Source: three-view drawing plus pictorial views. Frame: mm from the lowest corner of the part. Coordinates: 2 decimals unless noted, no trailing zeros. Order: outer loops, then holes, each group sorted by start corner. A loop starts at its lowest first (then second) coordinate and runs counter-clockwise, first axis right, second up. Notation, with made-up numbers: (21.25, 68.5) - (73.25, 68.5) arc R5 cw to (73.25, 73.5) - close; hole circle Ø3 at (71.25, 84.25). An arc over 180 degrees is marked (long way). Use a Markdown table: item, result. Add a question column.
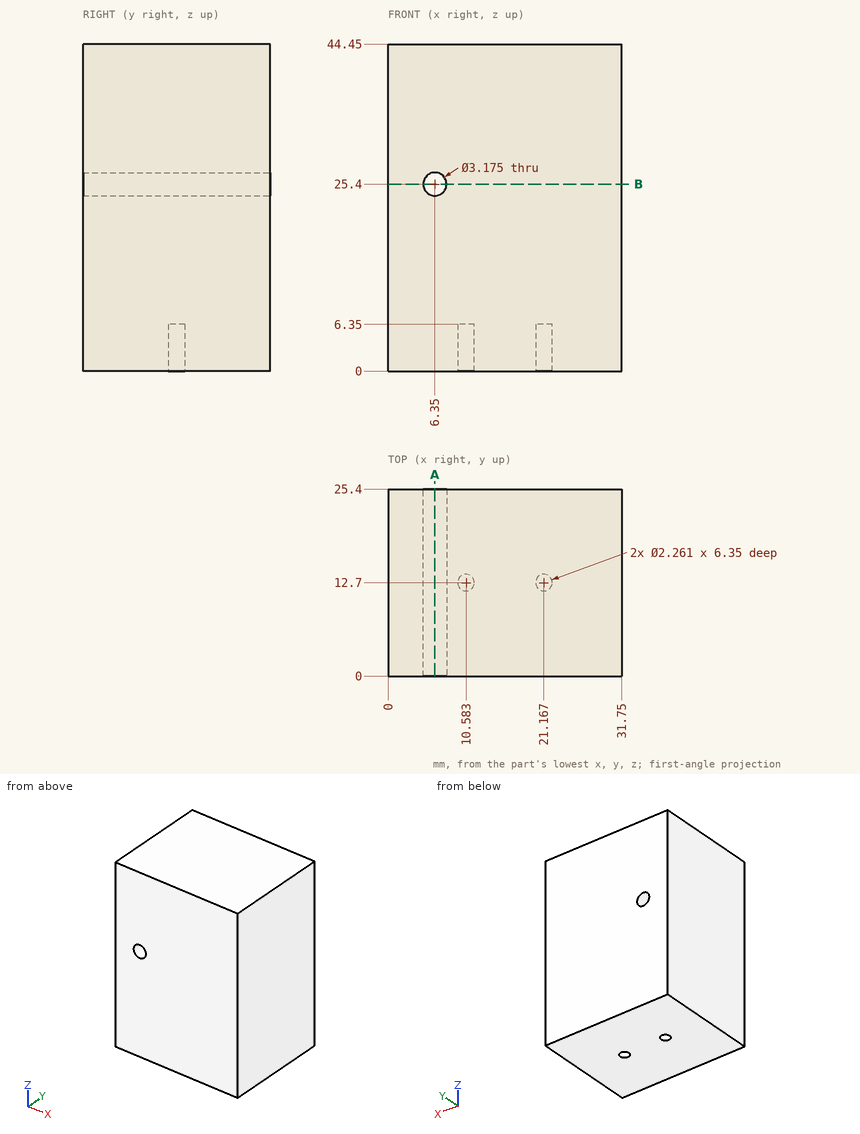
1) Section A-A (x = 6.35). Return loops of the section in (y, z).
2) Section B-B (z = 25.4). Return loops of the section in (x, y).
3) Ray query, line 1 along Z through (x, y) = (6.35, 13.75); line 2 along Z through (x, y) = (7, 5.5). Return the intervals inside material, ascending.
4) Pin query (flat end, axial travel): pin 1 (0.7 mm diameter, centred on x = 11, y = 13, fed in from -Z). Return the tip coordinate at first contact, or that it passes through.
Values follow:
| question | item | result |
|---|---|---|
| 1 | outline | (0, 0) - (25.4, 0) - (25.4, 23.81) - (0, 23.81) - close; (0, 26.99) - (25.4, 26.99) - (25.4, 44.45) - (0, 44.45) - close |
| 2 | outline | (0, 0) - (4.76, 0) - (4.76, 25.4) - (0, 25.4) - close; (7.94, 0) - (31.75, 0) - (31.75, 25.4) - (7.94, 25.4) - close |
| 3 | line 1 | z = 0 to 23.81, 26.99 to 44.45 |
| 3 | line 2 | z = 0 to 23.95, 26.85 to 44.45 |
| 4 | pin 1 | stops at z = 6.35 |
